For this review, take the finished solid that the model builds, in its own axes (mm). Face numbers are marked on the shaded views. A direction names the side the tool comes from. Round coordinates to 2 decimals unless told otherwise and drop trailing zeros. Order: outer loops, then holes, each group sorted by start corner. A loop starts at its lowest first (then second) coordinate and runs counter-clockwise, first axis right, second up. Notation, with made-up numbers: M 89,31.5 L 133,31.5 A22 ccw 133,66.5 Z; hole C 8,25.5 d4. An arc over 180 degrees is marked long. Answer as a JSON object with one key per item and string values.
from build123d import *

# Parameters (mm, degrees)
F0_R     = 6.2
F1_DEPTH = 2
F0_R_2   = 5.2
F2_DEPTH = 10
F3_R     = 1.25
F4_DEPTH = 15


with BuildPart() as f1:
    # F0 (on Front) → F1 (new body)
    with BuildSketch(Plane.XZ):
        with BuildLine():
            Line((1.2499564027, -8.2104398957), (6.7196736159, -8.2104398957))
            Line((6.7196736159, -8.2104398957), (6.7196736159, 8.2104398957))
            Line((6.7196736159, 8.2104398957), (1.2499564027, 8.2104398957))
            ThreePointArc((1.2499564027, 8.2104398957), (1.2499891006, 8.2052199934), (1.25, 8.2))
            ThreePointArc((1.25, 8.2), (-0.0052199934, 6.9500108994), (-1.2499564027, 8.2104398957))
            Line((-1.2499564027, 8.2104398957), (-6.7196736159, 8.2104398957))
            Line((-6.7196736159, 8.2104398957), (-6.7196736159, -8.2104398957))
            Line((-6.7196736159, -8.2104398957), (-1.2499564027, -8.2104398957))
            ThreePointArc((-1.2499564027, -8.2104398957), (-0.0052199934, -6.9500108994), (1.25, -8.2))
            ThreePointArc((1.25, -8.2), (1.2499891006, -8.2052199934), (1.2499564027, -8.2104398957))
        make_face()
        Circle(F0_R, mode=Mode.SUBTRACT)
        with BuildLine():
            Line((1.2499564027, 8.2104398957), (6.7196736159, 8.2104398957))
            Line((6.7196736159, 8.2104398957), (6.7196736159, 9.95100941))
            ThreePointArc((6.7196736159, 9.95100941), (0, 12.0439815451), (-6.7196736159, 9.95100941))
            Line((-6.7196736159, 9.95100941), (-6.7196736159, 8.2104398957))
            Line((-6.7196736159, 8.2104398957), (-1.2499564027, 8.2104398957))
            ThreePointArc((-1.2499564027, 8.2104398957), (0, 9.45), (1.2499564027, 8.2104398957))
        make_face()
        with BuildLine():
            Line((6.7196736159, -9.95100941), (6.7196736159, -8.2104398957))
            Line((6.7196736159, -8.2104398957), (1.2499564027, -8.2104398957))
            ThreePointArc((1.2499564027, -8.2104398957), (0, -9.45), (-1.2499564027, -8.2104398957))
            Line((-1.2499564027, -8.2104398957), (-6.7196736159, -8.2104398957))
            Line((-6.7196736159, -8.2104398957), (-6.7196736159, -9.95100941))
            ThreePointArc((-6.7196736159, -9.95100941), (0, -12.0439815451), (6.7196736159, -9.95100941))
        make_face()
    extrude(amount=F1_DEPTH)

    # F0 (on Front) → F2 (join)
    with BuildSketch(Plane.XZ):
        Circle(F0_R)
        Circle(F0_R_2, mode=Mode.SUBTRACT)
    extrude(amount=F2_DEPTH)

    # F3 (on face) → F4 (cut)
    with BuildSketch(Plane.YZ.offset(6.7196736159)):
        with Locations((-6, 0)):
            Circle(F3_R)
    extrude(amount=-F4_DEPTH, mode=Mode.SUBTRACT)


solid = f1.part
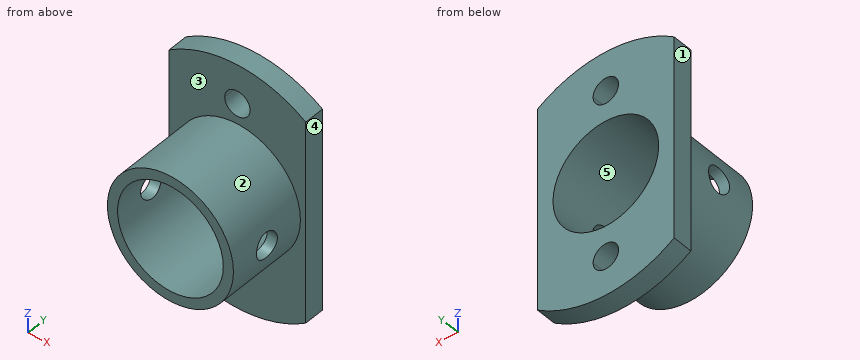
1) Add section D-D on y = -1.5. State how many separate pieces and enclosed holes the cut face has, and give its area (3 significant figures).
Geometry check:
{"separate pieces": "1", "enclosed holes": "3", "area": "211 mm²"}
2) For L1, parallel to Z at x = 0, y = -3; L2, parallel to Y at x = 5.9, z = 0, list the stretches that pass through material, from the lowest coordinate up.
Geometry check:
{"L1": "z = -6.2 to -5.2, 5.2 to 6.2", "L2": "y = -10 to -7.25, -4.75 to 0"}
3) Add section A-A on x = 0. State the section outline as (y, z) points.
Geometry check:
{"outline": "M -10,-6.2 L -2,-6.2 L -2,-6.95 L 0,-6.95 L 0,-5.2 L -10,-5.2 Z; M -10,5.2 L 0,5.2 L 0,6.95 L -2,6.95 L -2,6.2 L -10,6.2 Z; M -2,-12.04 L 0,-12.04 L 0,-9.45 L -2,-9.45 Z; M -2,9.45 L 0,9.45 L 0,12.04 L -2,12.04 Z"}
4) Machinability: for the marked faces 1 and 2, which of the approach directions +Z, -Z, +X, -X, +Y, -Y give a long, thin tool a straight path to every point of the face, cutting with its end or side? Answer none if there is none.
Geometry check:
{"face 1": "+Z, -Z, -X, +Y, -Y", "face 2": "-Y"}
5) Add section C-C on x = -4.25. State the section outline as (y, z) points.
Geometry check:
{"outline": "M -10,-4.51 L -2,-4.51 L -2,-11.25 L 0,-11.25 L 0,-3 L -10,-3 Z; M -10,3 L 0,3 L 0,11.25 L -2,11.25 L -2,4.51 L -10,4.51 Z"}
6) Insertion check: P1, Ø4, axis at x = -5, y = -5.5, coming from the +Z side; P2, Ø1.5, axis at x = -3.5, y = -8, coming from the +Z side; P3, Ø2, axis at x = 1, z = -7.5, coming from the +Y side; P4, Ø1, axis at y = -6, z = 2.5, coming from the +X side. Each pin has a flat end and moves straight along its axis. Give the tip position at first contact, or say it passes through.
Geometry check:
{"P1": "stops at z = 5.43", "P2": "stops at z = 5.56", "P3": "stops at y = 0", "P4": "stops at x = 5.87"}
7) Add section B-B on z = 0. State the section outline as (x, y) points.
Geometry check:
{"outline": "M -6.72,-2 L -6.2,-2 L -6.2,-4.75 L -5.2,-4.75 L -5.2,0 L -6.72,0 Z; M -6.2,-10 L -5.2,-10 L -5.2,-7.25 L -6.2,-7.25 Z; M 5.2,-10 L 6.2,-10 L 6.2,-7.25 L 5.2,-7.25 Z; M 5.2,-4.75 L 6.2,-4.75 L 6.2,-2 L 6.72,-2 L 6.72,0 L 5.2,0 Z"}
8) Mouldability with a two-part tool opening along X and no side actions: class the marked faces 3, 4 and 5 as +X half, -X half, draft (parallel to the pull), parting line (faces both ways), or undercut.
Geometry check:
{"face 3": "draft", "face 4": "+X half", "face 5": "undercut"}
